from build123d import *

# Parameters (mm, degrees)
F1_DEPTH      = 50.8
F1_DEPTH_BACK = 50.8
F2_R          = 9.849318
F3_DEPTH      = 214.428754
F4_W          = 201.727754
F4_H          = 88.9
F5_DEPTH      = 79.751232


with BuildPart() as f1:
    # F0 (on Front) → F1 (new body, two sides)
    with BuildSketch(Plane.XZ) as f1_sk:
        Polygon((-107.213877, 0), (0, 0), (107.213877, 0), (107.213877, 79.750232), (60.032729, 79.750232), (60.032729, 55.455457), (0, 55.455457), (-60.032729, 55.455457), (-60.032729, 79.750232), (-107.213877, 79.750232), align=None)
    extrude(amount=F1_DEPTH)
    extrude(f1_sk.sketch, amount=-F1_DEPTH_BACK)

    # F2 (on face) → F3 (cut, through all)
    with BuildSketch(Plane.YZ.offset(107.213877)):
        with Locations((0, 39.875116)):
            Circle(F2_R)
    extrude(amount=-F3_DEPTH, mode=Mode.SUBTRACT)

    # F4 (on face) → F5 (cut, through all)
    with BuildSketch(Plane(origin=(0, 0, 0), x_dir=(1, 0, 0), z_dir=(0, 0, -1))):
        Rectangle(F4_W, F4_H)
    extrude(amount=-F5_DEPTH, mode=Mode.SUBTRACT)


solid = f1.part
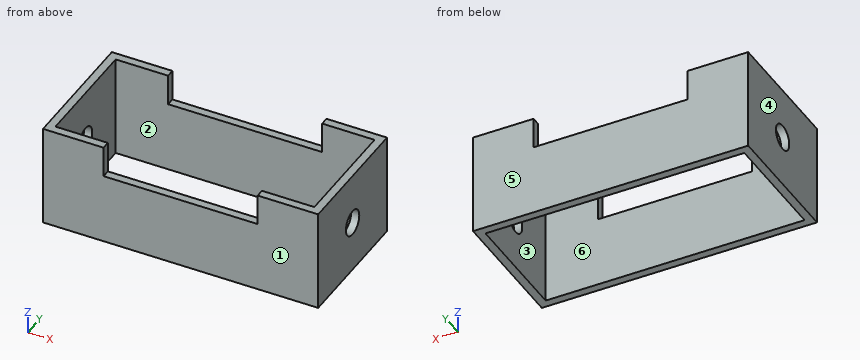
Could you check a few things on this model? Use its own coordinates, in mm. Face numbers are marked on the shaded views. A direction names the side the tool comes from. Coordinates: 2 decimals unless noted, no trailing zeros. Loops run counter-clockwise (first coordinate to the right, second up) from the corner with the lowest first, then second, coordinate; pieces in that order, holes last.
1. I need wall thicknesses on L1, parallel to Y at x = -94, z = 38.5; L2, parallel to X at y = -38.5, z = 12; L3, parallel to Z at x = -102.75, y = 0. Which ranges of each line are inside material? Lowest first, please.
2. Imagine slicing it at B-B (x = -10.5). Please give me the cut outline in (y, z), and give its area (3 significant figures).
3. For P1, Ø1.9, axis at x = 4, y = 47.5, coming from the +Z side; P2, Ø8, axis at x = 61, y = -38.5, coming from the -Z side; P3, Ø22.5, axis at y = 0, z = 39.88, coming from the +X side, each with a flat end and sliding along its axis, tell me the tip position at first contact or that it passes through.
4. Imagine slicing it at D-D (z = 36.5). Please give me the cut outline in (x, y).
5. Imagine slicing it at A-A (y = -27). Please give me the cut outline in (x, z), and give its area (3 significant figures).
6. We'd pull the mould along X, two halves only. Please class the marked faces 1, 2, 3 and 4: released by +X, released by -X, zero draft, split by the parting line, or undercut.
7. For the marked faces 5 and 6, which set-ups out of +Z, -Z, +X, -X, +Y, -Y let a thin tool reach every point of the face, with its end or its side?
8. Imagine slicing it at C-C (y = 0). Please give me the cut outline in (x, z), and give its area (3 significant figures).
Computed values:
1. L1: y = -50.8 to -44.45, 44.45 to 50.8
1. L2: x = -107.21 to -100.86, 100.86 to 107.21
1. L3: z = 0 to 30.03, 49.72 to 79.75
2. outline: (-50.8, 0) - (-44.45, 0) - (-44.45, 55.46) - (-50.8, 55.46) - close; (44.45, 0) - (50.8, 0) - (50.8, 55.46) - (44.45, 55.46) - close
2. area: 704 mm2
3. P1: stops at z = 55.46
3. P2: passes through
3. P3: stops at x = 107.21
4. outline: (-107.21, -50.8) - (107.21, -50.8) - (107.21, -9.25) - (100.86, -9.25) - (100.86, -44.45) - (-100.86, -44.45) - (-100.86, -9.25) - (-107.21, -9.25) - close; (-107.21, 9.25) - (-100.86, 9.25) - (-100.86, 44.45) - (100.86, 44.45) - (100.86, 9.25) - (107.21, 9.25) - (107.21, 50.8) - (-107.21, 50.8) - close
5. outline: (-107.21, 0) - (-100.86, 0) - (-100.86, 79.75) - (-107.21, 79.75) - close; (100.86, 0) - (107.21, 0) - (107.21, 79.75) - (100.86, 79.75) - close
5. area: 1,010 mm2
6. face 1: zero draft
6. face 2: undercut
6. face 3: undercut
6. face 4: released by -X
7. face 5: +Z, -Z, +X, -X, +Y
7. face 6: +Z, -Z
8. outline: (-107.21, 0) - (-100.86, 0) - (-100.86, 30.03) - (-107.21, 30.03) - close; (-107.21, 49.72) - (-100.86, 49.72) - (-100.86, 79.75) - (-107.21, 79.75) - close; (100.86, 0) - (107.21, 0) - (107.21, 30.03) - (100.86, 30.03) - close; (100.86, 49.72) - (107.21, 49.72) - (107.21, 79.75) - (100.86, 79.75) - close
8. area: 763 mm2
